```python
from build123d import *

# Parameters (mm, degrees)
SKETCH_1_W          = 125
SKETCH_1_H          = 85
EXTRUDE_1_DEPTH     = 1.5
SKETCH_2_W          = 98.3
SKETCH_2_H          = 62
CUT_EXTRUDE_1_DEPTH = 1.5
SKETCH_4_R          = 1.75
CUT_EXTRUDE_2_DEPTH = 10
SKETCH_5_R          = 1.75
CUT_EXTRUDE_3_DEPTH = 10
SKETCH_6_W          = 17
SKETCH_6_H          = 9
CUT_EXTRUDE_4_DEPTH = 10


with BuildPart() as part:
    # 스케치1 → 보스-돌출1 (new body)
    with BuildSketch(Plane(origin=(0, 0, 0), x_dir=(1, 0, 0), z_dir=(0, 1, 0))):
        with Locations((-7.35, 0)):
            Rectangle(SKETCH_1_W, SKETCH_1_H)
    extrude(amount=EXTRUDE_1_DEPTH)

    # 스케치2 → 컷-돌출1 (cut)
    with BuildSketch(Plane(origin=(0, 1.5, 0), x_dir=(1, 0, 0), z_dir=(0, 1, 0))):
        Rectangle(SKETCH_2_W, SKETCH_2_H)
    extrude(amount=-CUT_EXTRUDE_1_DEPTH, mode=Mode.SUBTRACT)

    # 스케치4 → 컷-돌출2 (cut)
    with BuildSketch(Plane(origin=(0, 1.5, 0), x_dir=(1, 0, 0), z_dir=(0, 1, 0))):
        with Locations((-61.07, 40)):
            Circle(SKETCH_4_R)
        with Locations((48.93, 40)):
            Circle(SKETCH_4_R)
        with Locations((48.93, -40)):
            Circle(SKETCH_4_R)
        with Locations((-61.07, -40)):
            Circle(SKETCH_4_R)
    extrude(amount=-CUT_EXTRUDE_2_DEPTH, mode=Mode.SUBTRACT)

    # 스케치5 → 컷-돌출3 (cut)
    with BuildSketch(Plane(origin=(0, 1.5, 0), x_dir=(1, 0, 0), z_dir=(0, 1, 0))):
        with Locations((-27.07, -40)):
            Circle(SKETCH_5_R)
        with Locations((14.93, -40)):
            Circle(SKETCH_5_R)
        with Locations((-27.07, 40)):
            Circle(SKETCH_5_R)
        with Locations((14.93, 40)):
            Circle(SKETCH_5_R)
    extrude(amount=-CUT_EXTRUDE_3_DEPTH, mode=Mode.SUBTRACT)

    # 스케치6 → 컷-돌출4 (cut)
    with BuildSketch(Plane.XZ):
        with Locations((-44.07, 40)):
            Rectangle(SKETCH_6_W, SKETCH_6_H)
        with Locations((31.93, 40)):
            Rectangle(SKETCH_6_W, SKETCH_6_H)
        with Locations((-44.07, -40)):
            Rectangle(SKETCH_6_W, SKETCH_6_H)
        with Locations((31.93, -40)):
            Rectangle(SKETCH_6_W, SKETCH_6_H)
    extrude(amount=-CUT_EXTRUDE_4_DEPTH, mode=Mode.SUBTRACT)


solid = part.part
```
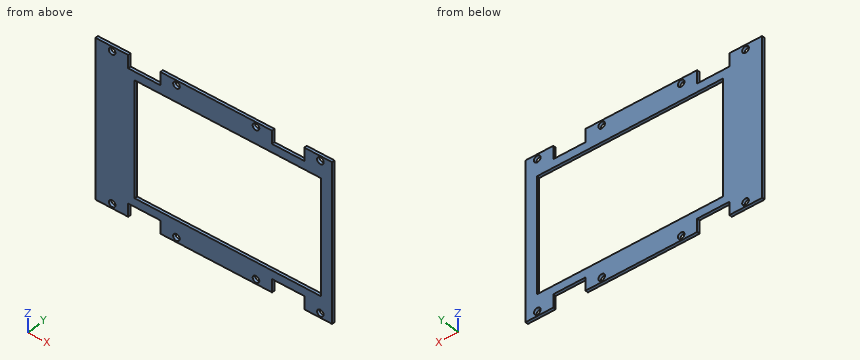
Geometry check sheet. Reference: the model listing, model coordinates, mm. Coordinates: 2 decimals unless noted, no trailing zeros. Order: outer loops, then holes, each group sorted by start corner. A loop starts at its lowest first (then second) coordinate and runs counter-clockwise, first axis right, second up. Notation, with made-up numbers: (32, 85) - (49, 85) arc R18 ccw to (49, 103) - close; hole circle Ø8 at (40.5, 35.5). An arc over 180 degrees is marked (long way). Answer in a Markdown table with one row per item. Add a question column.
1. Gauge pin test, flat end, axial feed: pin 1 Ø0.8 at (x, y) = (-42, 0.5) entering from +Z. Record the tip position at first contact, or that the pin passes through.
2. Section check B-B (x = -47.5). Enter the section's corners in (y, z).
3. Material ranges on L1, parallel to Z at x = 48.93, y = 0.7; L2, parallel to X at y = 0.75, z = -37.5; L3, parallel to Z at x = -8, y = 1.3, recorded low to high. Write a range as [from, to].
4. Section check D-D (x = 14.93). Enter the section's corners in (y, z), plus the area to 3 significant figures.
5. Section check C-C (y = 1.15). Give the number of separate pieces and of enclosed holes in the cut face, plus the area to 3 significant figures.
6. Section check A-A (z = 28). Enter the section's corners in (x, y), plus the area to 4 significant figures.
Data:
| question | item | result |
|---|---|---|
| 1 | pin 1 | stops at z = 35.5 |
| 2 | outline | (0, -35.5) - (1.5, -35.5) - (1.5, -31) - (0, -31) - close; (0, 31) - (1.5, 31) - (1.5, 35.5) - (0, 35.5) - close |
| 3 | L1 | z = [-42.5, -41.75], [-38.25, -31], [31, 38.25], [41.75, 42.5] |
| 3 | L2 | x = [-69.85, -52.57], [-35.57, 23.43], [40.43, 55.15] |
| 3 | L3 | z = [-42.5, -31], [31, 42.5] |
| 4 | outline | (0, -42.5) - (1.5, -42.5) - (1.5, -41.75) - (0, -41.75) - close; (0, -38.25) - (1.5, -38.25) - (1.5, -31) - (0, -31) - close; (0, 31) - (1.5, 31) - (1.5, 38.25) - (0, 38.25) - close; (0, 41.75) - (1.5, 41.75) - (1.5, 42.5) - (0, 42.5) - close |
| 4 | area | 24.0 mm² |
| 5 | separate pieces | 1 |
| 5 | enclosed holes | 9 |
| 5 | area | 3,980 mm² |
| 6 | outline | (-69.85, 0) - (-49.15, 0) - (-49.15, 1.5) - (-69.85, 1.5) - close; (49.15, 0) - (55.15, 0) - (55.15, 1.5) - (49.15, 1.5) - close |
| 6 | area | 40.05 mm² |
